Geometry check sheet. Reference: drawing and pictorial views, mm from the part's lowest x, y, z. Round coordinates to 2 decimals unless told otherwise and drop trailing zeros. Loops run counter-clockwise (first coordinate to the right, second up) from the corner with the lowest first, then second, coordinate; pieces in that order, holes last. Notation, with made-up numbers: (69.5, 32) - (105.5, 32) arc R7 cw to (105.5, 40) - close; hole circle Ø6 at (64.5, 37). An arc over 180 degrees is marked (long way). Answer in a Markdown table with one row per item. Add a question column.
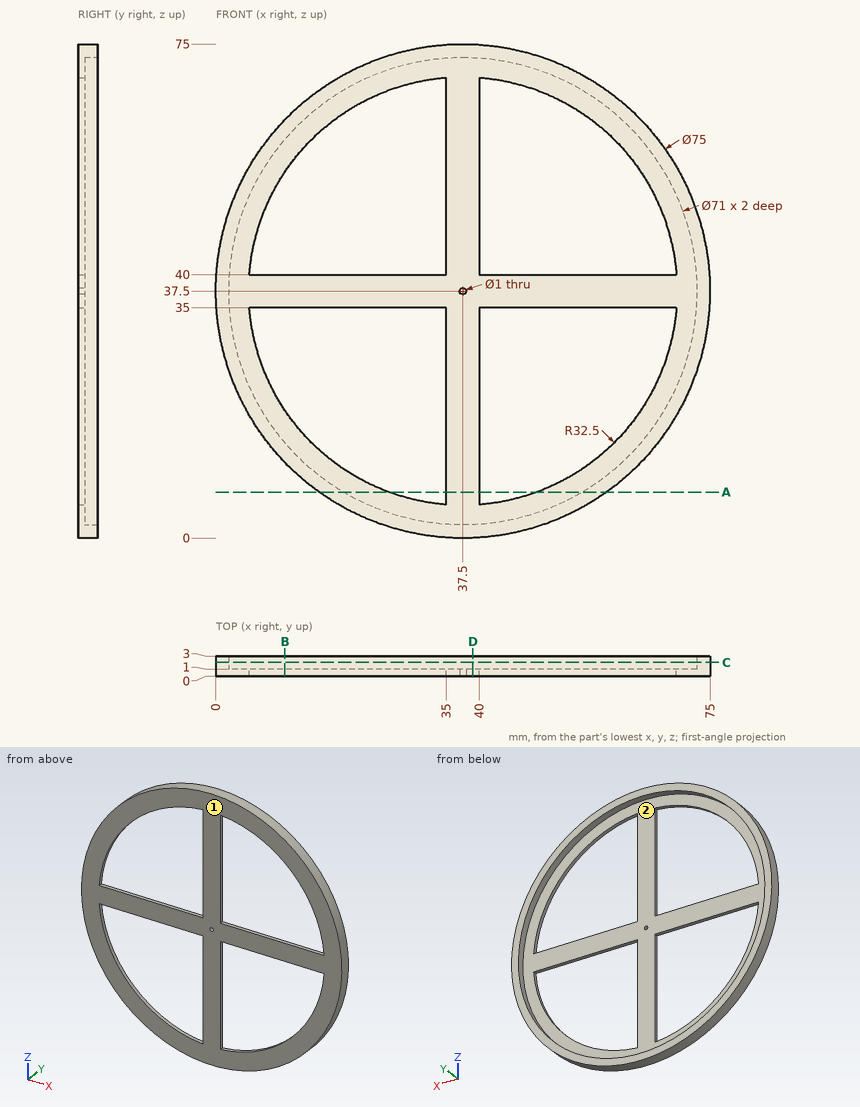
Q1. Cross-section at D-D, the plane x = 39. Enter the section's corners in (y, z), plus the area to 3 significant figures.
Q2. Scan lines: line 1 (X direction, y = 0.4, z = 37.5); line 2 (X direction, y = 0.85, z = 65); line 3 (Z direction, x = 49, y = 0.25). Record each from-to range of solid material in increasing order. Write a range as from..to.
Q3. Cross-section at C-C, the plane y = 2.05. Enter the section's corners in (x, z), plus the area to 3 significant figures.
Q4. Cross-section at B-B, the plane x = 10.5. Enter the section's corners in (y, z), plus the area to 3 significant figures.
Q5. Cross-section at A-A, the plane z = 7. Enter the section's corners in (x, y), plus the area to 3 significant figures.
Q6. Release check for a two-part mould opening along X. For the marked faces 1 and 2 record: +X half, -X half, draft (parallel to the pull), parting line (faces both ways), or undercut.
Q7. Depth check by flat-ended pin: P1, Ø2, axis at x = 18.5, z = 61.5, coming from the +Y side; P2, Ø8, axis at x = 53.5, z = 13.5, coming from the +Y side; P3, Ø0.8, axis at y = 0.5, z = 18, coming from the +X side; P4, Ø0.5, axis at x = 27, y = 0.5, coming from the -Z side. Enter the tip coordinate at first touch or a pass-through.
Check sheet entries:
| question | item | result |
|---|---|---|
| 1 | outline | (0, 0.03) - (3, 0.03) - (3, 2.03) - (1, 2.03) - (1, 72.97) - (3, 72.97) - (3, 74.97) - (0, 74.97) - close |
| 1 | area | 82.9 mm² |
| 2 | line 1 | 0..37, 38..75 |
| 2 | line 2 | 12..20.18, 35..40, 54.82..63 |
| 2 | line 3 | 1.81..7.1, 35..40, 67.9..73.19 |
| 3 | outline | circle Ø75 at (37.5, 37.5); hole circle Ø71 at (37.5, 37.5) |
| 3 | area | 459 mm² |
| 4 | outline | (0, 11.48) - (3, 11.48) - (3, 14.45) - (1, 14.45) - (1, 19.41) - (0, 19.41) - close; (0, 35) - (1, 35) - (1, 40) - (0, 40) - close; (0, 55.59) - (1, 55.59) - (1, 60.55) - (3, 60.55) - (3, 63.52) - (0, 63.52) - close |
| 4 | area | 32.8 mm² |
| 5 | outline | (15.68, 0) - (26.28, 0) - (26.28, 1) - (19.33, 1) - (19.33, 3) - (15.68, 3) - close; (35, 0) - (40, 0) - (40, 1) - (35, 1) - close; (48.72, 0) - (59.32, 0) - (59.32, 3) - (55.67, 3) - (55.67, 1) - (48.72, 1) - close |
| 5 | area | 40.8 mm² |
| 6 | face 1 | draft |
| 6 | face 2 | undercut |
| 7 | P1 | through |
| 7 | P2 | y = 1 |
| 7 | P3 | x = 69.77 |
| 7 | P4 | z = 1.43 |
